Model file for the job. Use its own axes, mm. A direction names the side the tool comes from. Give positions to 0.01 mm unless a question says otherwise; leave off trailing zeros. Write each loop counter-clockwise with the first axis right and the second up, starting at its lowest first coordinate (ties: lowest second). Pieces come first, ordered by that corner, then holes.
```python
from build123d import *

# Parameters (mm, degrees)
BOSS_EXTRUDE1_DEPTH = 62
SHELL1_T            = -6
FILLET2_R           = 10
FILLET3_R           = 10
SKETCH4_W           = 42.2
SKETCH4_H           = 27.964545036
CUT_EXTRUDE1_DEPTH  = 1.9
SKETCH5_R           = 25
CUT_EXTRUDE2_DEPTH  = 91.55523235
DRAFT1_ANGLE        = 56
SKETCH6_W           = 8
SKETCH6_H           = 46.353363522
SKETCH6_R           = 2.25
BOSS_EXTRUDE2_DEPTH = 5
FILLET4_R           = 5


with BuildPart() as part:
    # Sketch2 → Boss-Extrude1 (new body)
    with BuildSketch(Plane.XY):
        with BuildLine():
            Line((-40, 36.306779105), (-40, -36.306779105))
            ThreePointArc((-40, -36.306779105), (0, -52.5), (40, -36.306779105))
            Line((40, -36.306779105), (40, 36.306779105))
            ThreePointArc((40, 36.306779105), (0, 52.5), (-40, 36.306779105))
        make_face()
    extrude(amount=BOSS_EXTRUDE1_DEPTH)

    # Shell1
    shell1_openings = [part.faces().sort_by_distance(p)[0] for p in [
        (0, 0, 0),
    ]]
    offset(amount=SHELL1_T, openings=shell1_openings, kind=Kind.INTERSECTION)

    # Fillet2
    fillet2_edges = [part.edges().sort_by_distance(p)[0] for p in [
        (0, -52.5, 62),
        (40, 0, 62),
        (0, 52.5, 62),
        (40, 36.306779105, 31),
        (40, -36.306779105, 31),
        (-40, -36.306779105, 31),
        (-40, 36.306779105, 31),
        (-40, 0, 62),
    ]]
    fillet(fillet2_edges, radius=FILLET2_R)

    # Fillet3
    fillet3_edges = [part.edges().sort_by_distance(p)[0] for p in [
        (34, 33.681390875, 28),
        (-34, 33.681390875, 28),
        (-34, -33.681390875, 28),
        (34, -33.681390875, 28),
    ]]
    fillet(fillet3_edges, radius=FILLET3_R)

    # Sketch4 → Cut-Extrude1 (cut)
    with BuildSketch(Plane.XY):
        with Locations((0, -42.064156307)):
            Rectangle(SKETCH4_W, SKETCH4_H)
    extrude(amount=CUT_EXTRUDE1_DEPTH, mode=Mode.SUBTRACT)

    # Sketch5 → Cut-Extrude2 (cut, through all)
    with BuildSketch(Plane.XY.offset(62)):
        with Locations((0, 10.5)):
            Circle(SKETCH5_R)
    extrude(amount=-CUT_EXTRUDE2_DEPTH, mode=Mode.SUBTRACT)

    # Draft1
    draft1_faces = [part.faces().sort_by_distance(p)[0] for p in [
        (-25, 10.5, 59),
    ]]
    draft(draft1_faces, Plane(origin=(0, -5, 62), x_dir=(1, 0, 0), z_dir=(0, 0, 1)), DRAFT1_ANGLE)

    # Sketch6 → Boss-Extrude2 (add)
    # profile 1 of 2: a face of its own
    with BuildSketch(Plane.XY):
        with Locations((44, 0)):
            Rectangle(SKETCH6_W, SKETCH6_H)
        with Locations((44, 13.05590564)):
            Circle(SKETCH6_R, mode=Mode.SUBTRACT)
        with Locations((44, -13.05590564)):
            Circle(SKETCH6_R, mode=Mode.SUBTRACT)
    # profile 2 of 2: a face of its own
    with BuildSketch(Plane.XY):
        with Locations((-44, 0)):
            Rectangle(SKETCH6_W, SKETCH6_H)
        with Locations(Location((-44, -13.05590564, 0), (0, 0, 180))):
            Circle(SKETCH6_R, mode=Mode.SUBTRACT)
        with Locations(Location((-44, 13.05590564, 0), (0, 0, 180))):
            Circle(SKETCH6_R, mode=Mode.SUBTRACT)
    extrude(amount=BOSS_EXTRUDE2_DEPTH)

    # Fillet4
    fillet4_edges = [part.edges().sort_by_distance(p)[0] for p in [
        (48, -23.176681761, 2.5),
        (48, 23.176681761, 2.5),
        (-48, 23.176681761, 2.5),
        (-48, -23.176681761, 2.5),
    ]]
    fillet(fillet4_edges, radius=FILLET4_R)


solid = part.part
```
1. Which spindle directions (+Z, -Z, +X, -X, +Y, -Y) get a long thin tool onto all of the face, cutting with end or side? Do faces 1 (the flat face through (-36, 2, 0)), 2 (the flat face through (41, -23.177, 2)), 3 (the flat face through (44, 0, 5)), 4 (the cylindrical face through (-32.914, 33.389, 27.608)), 5 (the flat face through (48, 0, 2)). Say none if no direction does.
Calculated:
face 1: -Z, +X, -X, +Y, -Y
face 2: +Z, -Z, +X, -Y
face 3: +Z, +X, +Y, -Y
face 4: -Z
face 5: +Z, -Z, +X, +Y, -Y
2. Slice it at A-A, the plane y = -26.5. Write the cut outline in (x, z), and give its area (3 significant figures).
Calculated:
outline: (-40, 0) - (-34, 0) - (-34, 56) - (34, 56) - (34, 0) - (40, 0) - (40, 52) arc R10 ccw to (30, 62) - (-30, 62) arc R10 ccw to (-40, 52) - close
area: 1,110 mm2
3. Probe probe 1 along X at (y, z) = (-13, 3); probe 2 along X at (y, z) = (-20, 45.5); probe 3 along Y at (x, z) = (44, 3.6). List the from-to ranges inside material, lowest first.
Calculated:
probe 1: x = -48 to -46.25, -41.75 to -34, 34 to 41.75, 46.25 to 48
probe 2: x = -40 to -34, 34 to 40
probe 3: y = -23.08 to -15.31, -10.81 to 10.81, 15.31 to 23.08
4. Slice it at B-B, the plane x = 0. Write the cut outline in (y, z).
Calculated:
outline: (-52.5, 1.9) - (-46.5, 1.9) - (-46.5, 56) - (-5.6, 56) - (-14.5, 62) - (-42.5, 62) arc R10 ccw to (-52.5, 52) - close; (26.6, 56) - (46.5, 56) - (46.5, 0) - (52.5, 0) - (52.5, 52) arc R10 ccw to (42.5, 62) - (35.5, 62) - close
5. Pin check, flat tips, straight feed: P1, Ø6, axis at x = -3.5, z = 22, coming from the -Y side; P2, Ø9, axis at x = 45, y = 9, coming from the +Z side; P3, Ø1.5, axis at y = -10, z = 42, coming from the -X side. Stop position of each tip, or through.
Calculated:
P1: stops at y = -52.5
P2: stops at z = 5
P3: stops at x = -40
6. Pull direction Y, two halves, no side cores. Call faces 6 (the cylindrical face through (41.752, -12.957, 2.465)), 7 (the cylindrical face through (32.914, -33.389, 27.608)), 8 (the flat face through (0, -48, 1.9)), 9 (the flat face through (-42, 23.177, 2)): +Y half, -Y half, draft (parallel to the pull), parting line (faces both ways), or undercut.
Calculated:
face 6: undercut
face 7: undercut
face 8: draft
face 9: +Y half
